from build123d import *

# Parameters (mm, degrees)
SKETCH1_W           = 90
SKETCH1_H           = 110
SKETCH1_W_2         = 10
SKETCH1_H_2         = 40
SKETCH1_W_3         = 40
SKETCH1_H_3         = 10
BOSS_EXTRUDE1_DEPTH = 10
SKETCH2_R           = 4
CUT_EXTRUDE1_DEPTH  = 149.996644258
CUT_EXTRUDE2_DEPTH  = 149.996644258
SKETCH4_R           = 31.25
CUT_EXTRUDE3_DEPTH  = 3.5
SKETCH5_R           = 24.25
CUT_EXTRUDE4_DEPTH  = 149.802721749
SKETCH6_R           = 5
CUT_EXTRUDE5_DEPTH  = 149.996644258
SKETCH8_W           = 20
SKETCH8_H           = 5
SKETCH8_W_2         = 15
BOSS_EXTRUDE2_DEPTH = 10


with BuildPart() as part:
    # Sketch1 → Boss-Extrude1 (new body)
    with BuildSketch(Plane(origin=(0, 0, 0), x_dir=(1, 0, 0), z_dir=(0, 1, 0))):
        with Locations((45, 55)):
            Rectangle(SKETCH1_W, SKETCH1_H)
        with Locations((-5, 65)):
            Rectangle(SKETCH1_W_2, SKETCH1_H_2)
        with Locations((95, 65)):
            Rectangle(SKETCH1_W_2, SKETCH1_H_2)
        with Locations((45, -5)):
            Rectangle(SKETCH1_W_3, SKETCH1_H_3)
    extrude(amount=BOSS_EXTRUDE1_DEPTH)

    # Sketch2 → Cut-Extrude1 (cut, through all)
    with BuildSketch(Plane(origin=(0, 10, 0), x_dir=(1, 0, 0), z_dir=(0, 1, 0))):
        with Locations(Location((23.122776972, 102.57, 0), (0, 0, 270))):
            Circle(SKETCH2_R)
        with Locations((23.122776972, 120.41)):
            Circle(SKETCH2_R)
    extrude(amount=-CUT_EXTRUDE1_DEPTH, mode=Mode.SUBTRACT)

    # Sketch3 → Cut-Extrude2 (cut, through all)
    with BuildSketch(Plane(origin=(0, 10, 0), x_dir=(1, 0, 0), z_dir=(0, 1, 0))):
        with BuildLine():
            ThreePointArc((65.351977614, 81.42565129), (61.457970709, 79.741397678), (63.142224321, 75.847390774))
            Line((63.142224321, 75.847390774), (65.351977614, 81.42565129))
        make_face()
        with BuildLine():
            Line((65.351977614, 81.42565129), (63.142224321, 75.847390774))
            ThreePointArc((63.142224321, 75.847390774), (65.93312737, 76.155127276), (67.247100967, 78.636521032))
            ThreePointArc((67.247100967, 78.636521032), (66.728494723, 80.322547434), (65.351977614, 81.42565129))
        make_face()
        with BuildLine():
            ThreePointArc((58.722717735, 64.690869742), (61.513620784, 64.998606245), (62.827594381, 67.48))
            Line((62.827594381, 67.48), (59.827594381, 67.48))
            Line((59.827594381, 67.48), (58.722717735, 64.690869742))
        make_face()
        with BuildLine():
            Line((59.827594381, 67.48), (62.827594381, 67.48))
            ThreePointArc((62.827594381, 67.48), (62.308988137, 69.166026403), (60.932471028, 70.269130258))
            Line((60.932471028, 70.269130258), (59.827594381, 67.48))
        make_face()
        with BuildLine():
            Line((58.722717735, 64.690869742), (59.827594381, 67.48))
            Line((59.827594381, 67.48), (56.827594381, 67.48))
            ThreePointArc((56.827594381, 67.48), (57.346200626, 65.793973597), (58.722717735, 64.690869742))
        make_face()
        with BuildLine():
            Line((56.827594381, 67.48), (59.827594381, 67.48))
            Line((59.827594381, 67.48), (60.932471028, 70.269130258))
            ThreePointArc((60.932471028, 70.269130258), (58.141567979, 69.961393755), (56.827594381, 67.48))
        make_face()
    extrude(amount=-CUT_EXTRUDE2_DEPTH, mode=Mode.SUBTRACT)

    # Sketch4 → Cut-Extrude3 (cut)
    with BuildSketch(Plane(origin=(0, 10, 0), x_dir=(1, 0, 0), z_dir=(0, 1, 0))):
        with Locations(Location((36.72, 31.47, 0), (0, 0, 270))):
            Circle(SKETCH4_R)
    extrude(amount=-CUT_EXTRUDE3_DEPTH, mode=Mode.SUBTRACT)

    # Sketch5 → Cut-Extrude4 (cut, through all)
    with BuildSketch(Plane(origin=(0, 6.5, 0), x_dir=(1, 0, 0), z_dir=(0, 1, 0))):
        with Locations(Location((36.72, 31.47, 0), (0, 0, 270))):
            Circle(SKETCH5_R)
    extrude(amount=-CUT_EXTRUDE4_DEPTH, mode=Mode.SUBTRACT)

    # Sketch6 → Cut-Extrude5 (cut, through all)
    with BuildSketch(Plane(origin=(0, 10, 0), x_dir=(1, 0, 0), z_dir=(0, 1, 0))):
        with Locations((63.314917683, 111.209559188)):
            Circle(SKETCH6_R)
    extrude(amount=-CUT_EXTRUDE5_DEPTH, mode=Mode.SUBTRACT)

    # Sketch8 → Boss-Extrude2 (add)
    with BuildSketch(Plane(origin=(0, 0, -110), x_dir=(-1, 0, 0), z_dir=(0, 0, -1))):
        with Locations((-80, 2.5)):
            Rectangle(SKETCH8_W, SKETCH8_H)
        with Locations((-7.5, 2.5)):
            Rectangle(SKETCH8_W_2, SKETCH8_H)
        with Locations((-45, 2.5)):
            Rectangle(SKETCH8_W, SKETCH8_H)
    extrude(amount=BOSS_EXTRUDE2_DEPTH)


solid = part.part
Design review of the part built by this model. Coordinates are the model's own, in mm. A direction names the side the tool comes from. Round coordinates to 2 decimals unless told otherwise and drop trailing zeros. Loops run counter-clockwise (first coordinate to the right, second up) from the corner with the lowest first, then second, coordinate; pieces in that order, holes last. Notation, with made-up numbers: M 19.5,16 L 58.5,16 A30 cw 58.5,49 Z; hole C 32,54.25 d3. An arc over 180 degrees is marked long. Answer as a JSON object with one key per item and string values.
Item 1: Machinability: for faces 5 (the flat face through (95, 5, -85)), 6 (the flat face through (65, 5, 5)), 7 (the flat face through (0, 5, -22)), 8 (the flat face through (35, 2, -115)), which of the approach directions +Z, -Z, +X, -X, +Y, -Y give a long, thin tool a straight path to every point of the face, cutting with its end or side? Answer none if there is none.
Answer sheet:
{"face 5": "-Z, +X, +Y, -Y", "face 6": "+Z, +X, +Y, -Y", "face 7": "+Z, -X, +Y, -Y", "face 8": "-Z, +Y, -Y"}
Item 2: We need section A-A on z = -102.57. Give the boundary of the cut face in (x, y), and give its area (3 significant figures).
Answer sheet:
{"outline": "M 0,0 L 19.12,0 L 19.12,10 L 0,10 Z; M 27.12,0 L 90,0 L 90,10 L 27.12,10 Z", "area": "820 mm^2"}
Item 3: Clearance check with flat-ended pins moving along their axes: P1, Ø4, axis at y = 3, z = -113.5, coming from the +X side; P2, Ø3, axis at x = 4.5, z = -116, coming from the +Y side; P3, Ø2.5, axis at y = 2, z = -117, coming from the -X side. State where each tip first meets the part, or that it passes through.
Answer sheet:
{"P1": "stops at x = 90", "P2": "stops at y = 5", "P3": "stops at x = 0"}
Item 4: We need section B-B on x = 36.72. Give the boundary of the cut face in (y, z).
Answer sheet:
{"outline": "M 0,-120 L 5,-120 L 5,-110 L 10,-110 L 10,-62.72 L 6.5,-62.72 L 6.5,-55.72 L 0,-55.72 Z; M 0,-7.22 L 6.5,-7.22 L 6.5,-0.22 L 10,-0.22 L 10,10 L 0,10 Z"}
Item 5: Wall thickness on L1, parallel to X at y = 4.5, z = -31.47; L2, parallel to X at y = 8.6, z = -31.47; L3, parallel to Z at x = 22, y = 3.5: over which ranges is each line inside the solid? List them lowest first. Write a range as from..to.
Answer sheet:
{"L1": "x = 0..12.47, 60.97..90", "L2": "x = 0..5.47, 67.97..90", "L3": "z = -110..-106.41, -98.73..-50.74, -12.2..0"}
Item 6: The part is to be moulded in two halves that separate along Z. For faces 1 (the flat face through (45, 5, -115)), 2 (the cylindrical face through (15.206, 3.296, -20.28)), 3 (the flat face through (-5, 5, -85)), 4 (the cylindrical face through (67.704, 8.274, -35.538)), say which applies: pulls with the +Z half, pulls with the -Z half, needs draft (parallel to the pull), parting line crosses it, or undercut.
Answer sheet:
{"face 1": "needs draft", "face 2": "undercut", "face 3": "pulls with the -Z half", "face 4": "undercut"}
Item 7: We need section D-D on z = -31.47. Give the boundary of the cut face in (x, y).
Answer sheet:
{"outline": "M 0,0 L 12.47,0 L 12.47,6.5 L 5.47,6.5 L 5.47,10 L 0,10 Z; M 60.97,0 L 90,0 L 90,10 L 67.97,10 L 67.97,6.5 L 60.97,6.5 Z"}
Item 8: We need section C-C on y = 8.5. Give the boundary of the cut face in (x, z).
Answer sheet:
{"outline": "M -10,-85 L 0,-85 L 0,-110 L 58.46,-110 A5 cw 68.17,-110 L 90,-110 L 90,-85 L 100,-85 L 100,-45 L 90,-45 L 90,0 L 65,0 L 65,10 L 25,10 L 25,0 L 0,0 L 0,-45 L -10,-45 Z; hole C 36.72,-31.47 d62.5; hole C 23.12,-102.57 d8; hole C 59.83,-67.48 d6; hole C 64.25,-78.64 d6"}
